The drawing under review shows one solid part. Ordinate dimensions are in mm from its lowest x, y, z. A direction names the side the tool comes from. Coordinates: 2 decimals unless noted, no trailing zeros. Write each loop counter-clockwise with the first axis right and the second up, starting at its lowest first coordinate (ties: lowest second). Pieces come first, ordered by that corner, then holes.
Q1. Insertion check: pin 1 (6 mm diameter, centred on x = 56, y = 42.5, fed in from +Z); pin 2 (6 mm diameter, centred on y = 42, z = 69.5, fed in from +X); pin 3 (20 mm diameter, centred on y = 62.5, z = 39, fed in from +X). Each pin has a flat end and moves straight along its axis. Give the tip position at first contact, or say it passes through.
Q2. Take a section at B-B (y = 71). Give the boundary of the cut face in (x, z).
Q3. Take a section at A-A (z = 34). Give the boundary of the cut face in (x, y), and give its area (3 significant figures).
Q4. Mouldability with a two-part tool opening along Y and no side actions: class the marked faces 6, 7 and 8 as pulls with the +Y half, pulls with the -Y half, needs draft (parallel to the pull), parting line crosses it, or undercut.
Q5. Take a section at C-C (z = 19.5). Give the boundary of the cut face in (x, y), and give its area (3 significant figures).
Q6. Take a section at D-D (x = 38.5). Give the boundary of the cut face in (y, z), and give its area (3 significant figures).
Q7. For probe 1 along Y at (x, z) = (46.5, 43.5); probe 2 along Y at (x, z) = (36, 91.5); probe 3 along X at (y, z) = (40.5, 19), list the stretches that pass through material, from the lowest coordinate up.
Q8. Machinability: for the marked faces 1, 2, 3, 4 and 5, which of the approach directions +Z, -Z, +X, -X, +Y, -Y give a long, thin tool a straight path to every point of the face, cutting with its end or side? Answer none if there is none.
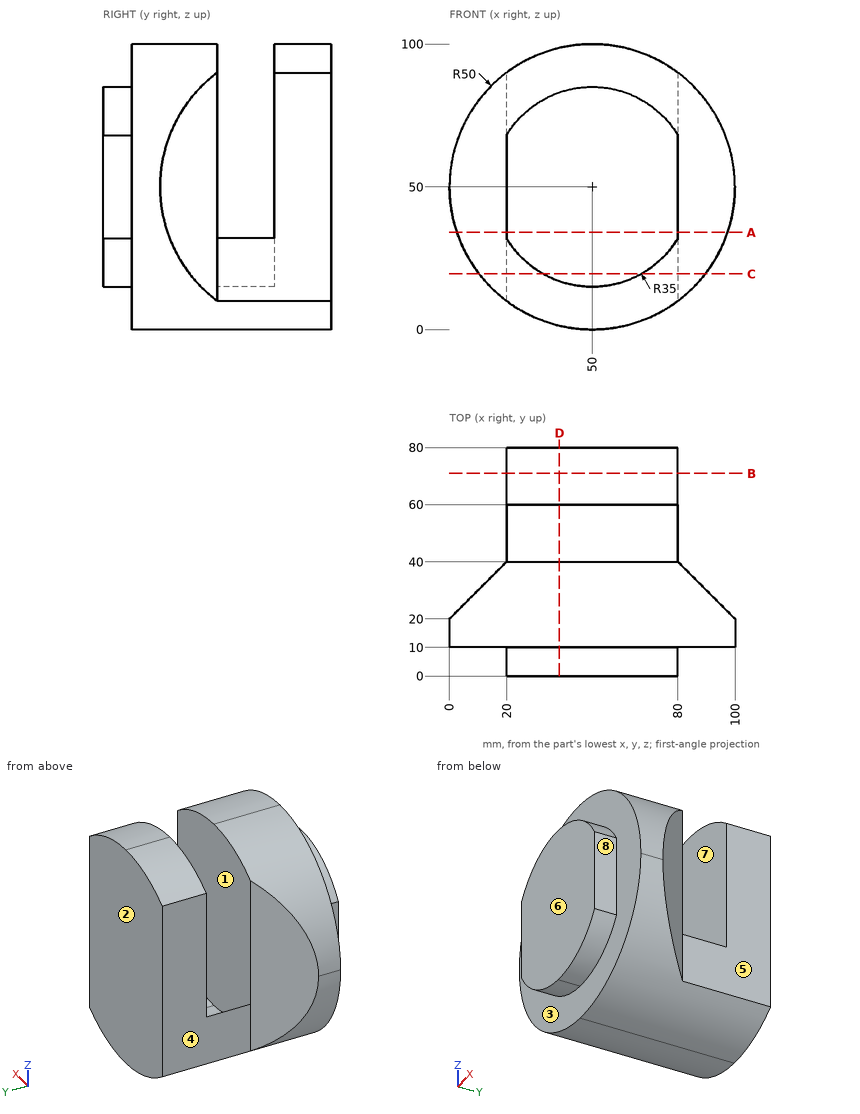
Response:
1. pin 1: stops at z = 99.81
1. pin 2: stops at x = 81
1. pin 3: stops at x = 80
2. outline: (20, 10) arc R50 ccw to (80, 10) - (80, 90) arc R50 ccw to (20, 90) - close
3. outline: (2.63, 10) - (20, 10) - (20, 0) - (80, 0) - (80, 10) - (97.37, 10) - (97.37, 22.63) - (80, 40) - (20, 40) - (2.63, 22.63) - close; (20, 60) - (80, 60) - (80, 80) - (20, 80) - close
3. area: 4,340 mm2
4. face 6: pulls with the -Y half
4. face 7: undercut
4. face 8: needs draft
5. outline: (10.38, 10) - (32.83, 10) - (32.83, 0) - (67.17, 0) - (67.17, 10) - (89.62, 10) - (89.62, 30.38) - (80, 40) - (80, 80) - (20, 80) - (20, 40) - (10.38, 30.38) - close; hole (32.83, 40) - (67.17, 40) - (67.17, 60) - (32.83, 60) - close
5. area: 4,340 mm2
6. outline: (0, 16.94) - (10, 16.94) - (10, 1.34) - (80, 1.34) - (80, 98.66) - (60, 98.66) - (60, 16.94) - (40, 16.94) - (40, 98.66) - (10, 98.66) - (10, 83.06) - (0, 83.06) - close
6. area: 5,840 mm2
7. probe 1: y = 0 to 40, 60 to 80
7. probe 2: y = 10 to 40, 60 to 80
7. probe 3: x = 20 to 33.75, 66.25 to 80
8. face 1: +Z
8. face 2: +Z, -Z, +X, -X, +Y
8. face 3: -Y
8. face 4: +Z, -Z, -X, +Y
8. face 5: +Z, -Z, +X, +Y
